Here's how the part is built. I have some questions about the finished solid (model axes, mm). Face numbers are marked on the shaded views. A direction names the side the tool comes from. Coordinates: 2 decimals unless noted, no trailing zeros. Order: outer loops, then holes, each group sorted by start corner. A loop starts at its lowest first (then second) coordinate and runs counter-clockwise, first axis right, second up. Notation, with made-up numbers: (6.5, 12.25) - (10.5, 12.25) arc R26 cw to (10.5, 48.25) - close; hole circle Ø1 at (12.5, 22). An arc over 180 degrees is marked (long way). Use one line per item in the form item = value. Start each with the question number.
from build123d import *

# Parameters (mm, degrees)
F1_DEPTH = 127
F2_DEPTH = 3.175
F3_W     = 101.6
F3_H     = 101.6
F4_DEPTH = 0.508
F6_DEPTH = 12.7
F7_R     = 7.62


with BuildPart() as f1:
    # F0 (on Top) → F1 (new body)
    with BuildSketch(Plane.XY):
        Polygon((-53.975, -56.026683), (0, -56.026683), (53.975, -56.026683), (53.975, 51.923317), (-53.975, 51.923317), align=None)
        Polygon((50.8, -52.851683), (0, -52.851683), (-50.8, -52.851683), (-50.8, 48.748317), (50.8, 48.748317), align=None, mode=Mode.SUBTRACT)
    extrude(amount=F1_DEPTH)

    # F0 (on Top) → F2 (join)
    with BuildSketch(Plane.XY):
        Polygon((-50.8, -52.851683), (0, -52.851683), (50.8, -52.851683), (50.8, 48.748317), (-50.8, 48.748317), align=None)
    extrude(amount=F2_DEPTH)

    # F3 (on face) → F4 (join)
    with BuildSketch(Plane.XY.offset(127)):
        with Locations((0, -2.051683)):
            Rectangle(F3_W, F3_H)
    extrude(amount=-F4_DEPTH)

    # F5 (on face) → F6 (cut)
    with BuildSketch(Plane.XY.offset(127)):
        with BuildLine():
            add(Edge.make_bspline(
                [(44.45, 0), (44.45, 58.29217), (-22.225, 29.146085), (-88.9, 0), (-22.225, -29.146085), (44.45, -58.29217), (44.45, 0)],
                knots=[0, 0, 0, 2.094395, 2.094395, 4.18879, 4.18879, 6.283185, 6.283185, 6.283185], degree=2, weights=[1, 0.5, 1, 0.5, 1, 0.5, 1]))
        make_face()
    extrude(amount=-F6_DEPTH, mode=Mode.SUBTRACT)

    # F7
    f7_edges = [f1.edges().sort_by_distance(p)[0] for p in [
        (-53.975, -56.026683, 63.5),
        (-53.975, 51.923317, 63.5),
        (53.975, 51.923317, 63.5),
        (53.975, -56.026683, 63.5),
    ]]
    fillet(f7_edges, radius=F7_R)


solid = f1.part
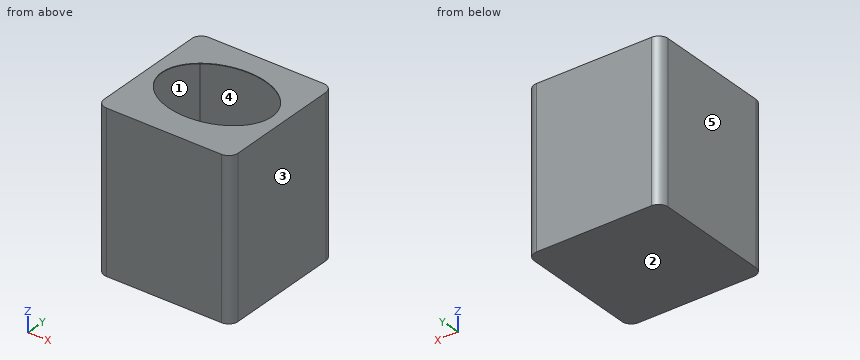
1) If we mould it in two halves opening along Z, with no side actions, what happens to the marked faces 1, 2 and 3? For each: pulls with the +Z half, pulls with the -Z half, needs draft (parallel to the pull), parting line crosses it, or undercut.
2) For pin 1 (5 mm diameter, centred on x = -34, y = 3.5, fed in from +Z) (3 decimals), with a flat end and sliding along its axis, tell me the tip position at first contact or that it passes through.
3) Suppose I cut it at B-B, the plane z = 85. List the corners of the cut face in (x, y) for me (3 decimals), then the cut area to 3 significant figures.
4) Which directions (+Z, -Z, +X, -X, +Y, -Y) give clear straight access to the entire face, cutting with the end or side of a thin tool? Please do the marked faces 4 and 5.
5) I need wall thicknesses on probe 1 along Y at (x, z) = (0, 101.5); probe 2 along X at (y, z) = (22.5, 51) (3 decimals); probe 3 along Z at (x, y) = (-40, -46.5) (3 decimals). Which ranges of each line are inside material? Lowest first, please. Write a range as [from, to].
6) Suppose I cut it at A-A, the plane y = 37.5. List the corners of the cut face in (x, z) for me (3 decimals), then the cut area to 3 significant figures.
From the geometry:
q1.face_1 = undercut
q1.face_2 = pulls with the -Z half
q1.face_3 = needs draft
q2.pin_1 = 3.175
q3.outline = (-53.975, -48.407) arc R7.62 ccw to (-46.355, -56.027) - (46.355, -56.027) arc R7.62 ccw to (53.975, -48.407) - (53.975, 44.303) arc R7.62 ccw to (46.355, 51.923) - (-46.355, 51.923) arc R7.62 ccw to (-53.975, 44.303) - close; hole (-50.8, -52.852) - (50.8, -52.852) - (50.8, 48.748) - (-50.8, 48.748) - close
q3.area = 1,280 mm2
q4.face_4 = none
q4.face_5 = +Z, -Z, -X, +Y, -Y
q5.probe_1 = [-56.03, -52.85], [48.75, 51.92]
q5.probe_2 = [-53.975, -50.8], [50.8, 53.975]
q5.probe_3 = [0, 3.175], [126.492, 127]
q6.outline = (-53.975, 0) - (53.975, 0) - (53.975, 127) - (-53.975, 127) - close; hole (-50.8, 3.175) - (50.8, 3.175) - (50.8, 126.492) - (-50.8, 126.492) - close
q6.area = 1,180 mm2
